```python
from build123d import *
from build123d.topology import SkipClean

# Parameters (mm, degrees)
BOSS_EXTRUDE1_DEPTH      = 10
BOSS_EXTRUDE1_DEPTH_BACK = 5
SKETCH1_R                = 25
CUT_EXTRUDE1_DEPTH       = 5
BOSS_EXTRUDE2_DEPTH      = 5


with BuildPart() as part:
    # Sketch1 → Boss-Extrude1 (new, two sides: drawn at the far end of the back side and taken through both)
    with BuildSketch(Plane(origin=(0, 0, 0), x_dir=(0, 0, -1), z_dir=(1, 0, 0)).offset(-BOSS_EXTRUDE1_DEPTH_BACK)):
        Circle(SKETCH1_R)
    extrude(amount=BOSS_EXTRUDE1_DEPTH + BOSS_EXTRUDE1_DEPTH_BACK)

    # Sketch2 → Cut-Extrude1 (cut)
    with BuildSketch(Plane(origin=(10, 0, 0), x_dir=(0, 0, -1), z_dir=(1, 0, 0))):
        with BuildLine():
            Line((2.5, 24.874685928), (2.5, -24.874685928))
            ThreePointArc((2.5, -24.874685928), (0, -25), (-2.5, -24.874685928))
            Line((-2.5, -24.874685928), (-2.5, 24.874685928))
            ThreePointArc((-2.5, 24.874685928), (0, 25), (2.5, 24.874685928))
        make_face()
    extrude(amount=-CUT_EXTRUDE1_DEPTH, mode=Mode.SUBTRACT)

    # Sketch4 → Boss-Extrude2 (add)
    with SkipClean():  # the faces are left unmerged after this step: merging them gives an invalid solid
        with BuildSketch(Plane.ZY.offset(5)):
            with BuildLine():
                Line((-24.874685928, -2.5), (24.874685928, -2.5))
                ThreePointArc((24.874685928, -2.5), (25, 0), (24.874685928, 2.5))
                Line((24.874685928, 2.5), (-24.874685928, 2.5))
                ThreePointArc((-24.874685928, 2.5), (-25, 0), (-24.874685928, -2.5))
            make_face()
        extrude(amount=BOSS_EXTRUDE2_DEPTH)


solid = part.part
```
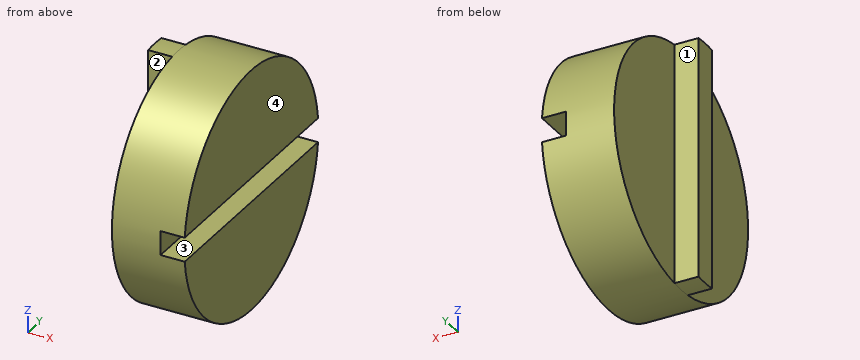
Could you check a few things on this model? Use its own coordinates, in mm. Face numbers are marked on the shaded views. A direction names the side the tool comes from. Round coordinates to 2 decimals unless told otherwise and drop trailing zeros. Order: outer loops, then holes, each group sorted by start corner. A loop starts at its lowest first (then second) coordinate and runs counter-clockwise, first axis right, second up. Notation, with made-up numbers: M 63,-31.75 L 74,-31.75 A26 cw 74,-13.75 Z; hole C 21,36 d1. An arc over 180 degrees is marked long. One line per question, with ' | ' between items. Start each with the question number.
(1) For the marked faces 1, 2, 3 and 4, which set-ups out of +Z, -Z, +X, -X, +Y, -Y let a thin tool reach every point of the face, with its end or its side?
(2) Suppose I cut it at D-D on x = -7.5. List the corners of the cut face in (y, z) for me.
(3) Suppose I cut it at B-B on z = 0. List the corners of the cut face in (x, y) for me, then the cut area to 3 significant figures.
(4) Please list where these lines run through material, in increasing order: line 1 along Z through (x, y) = (-5.25, 0); line 2 along X through (y, z) = (3.5, 5); line 3 along Y through (x, z) = (-7, -11).
(5) Suppose I cut it at A-A on y = 0. List the corners of the cut face in (x, z) for me.
(6) Suppose I cut it at C-C on x = 7. List the corners of the cut face in (y, z) for me.
(7) For P1, Ø1.5, axis at y = -3, z = -0.5, coming from the +X side; P2, Ø7, axis at y = 15, z = 9, coming from the -X side; P3, Ø4, axis at x = -6.5, z = -3, coming from the +Y side, each with a flat end and sliding along its axis, tell me the tip position at first contact or that it passes through.
Geometry results:
1) face 1: +Z, -Z, -X, +Y | face 2: +Z, -Z, -X, -Y | face 3: +X, +Y, -Y | face 4: +Z, -Z, +X, +Y, -Y
2) outline: M -2.5,-24.87 A25 ccw 2.5,-24.87 L 2.5,24.87 A25 ccw -2.5,24.87 Z
3) outline: M -10,-2.5 L -5,-2.5 L -5,-25 L 5,-25 L 5,25 L -5,25 L -5,2.5 L -10,2.5 Z | area: 525 mm²
4) line 1: -25 to 25 | line 2: -5 to 10 | line 3: -2.5 to 2.5
5) outline: M -10,-25 L 10,-25 L 10,-2.5 L 5,-2.5 L 5,2.5 L 10,2.5 L 10,25 L -10,25 Z
6) outline: M -24.87,-2.5 A25 ccw 24.87,-2.5 Z; M -24.87,2.5 L 24.87,2.5 A25 ccw Z
7) P1: x = 5 | P2: x = -5 | P3: y = 24.94
